Input: part model. Units: mm. Frame: model coordinates. A direction names the side the tool comes from. Coordinates: 2 decimals unless noted, no trailing zeros. Write each loop counter-clockwise with the first axis right and the second up, starting at its lowest first coordinate (ties: lowest second). Pieces come first, ordered by that corner, then holes. Notation, with made-up numbers: (19.25, 36.5) - (57.25, 36.5) arc R24 ccw to (57.25, 53.5) - close; hole circle Ø8 at (55.25, -17). An arc over 180 degrees is marked (long way). One line per question, with ' | ' between items. Start each with the question number.
1) Section query C-C on x = -10. Return loops of the section in (y, z).
2) Section query A-A on x = 0. Return loops of the section in (y, z).
3) Line query: line 1 (X direction, y = -25.95, z = -6.25); line 2 (X direction, y = 10.5, z = 16); line 3 (X direction, y = 39, z = -12.5). Output: solid intervals per line, ascending.
4) Section query B-B on z = 0. Return loops of the section in (x, y), and give its area (3 significant figures).
5) Draft query along X for faces 1 (the flat face through (8.35, 1.67, -7.66)), 2 (the flat face through (-1.4, -25, 11.2)), 3 (the flat face through (0, -28, 0)). Return one class per face: released by +X, released by -X, zero draft, split by the parting line, or undercut.
6) First-contact query: P1, Ø3.5, axis at x = -10, y = 3.5, coming from the +Z side; P2, Ø3, axis at x = 8.5, y = 34, coming from the -Z side; P3, Ø10, axis at y = -17, z = 6, coming from the -X side. Flat tips, straight axial feed; report the tip coordinate or a pass-through.
7) Reachability of faces 4 (the cylindrical face through (0.526, -26.479, 14.169)), 5 (the flat face through (-2.46, -9.28, 13.94)) from +Z, -Z, +X, -X, +Y, -Y: full face, straight path, thin tool, end or side. Return the list, or none.
```python
from build123d import *

# Parameters (mm, degrees)
SKETCH_1_R                  = 20.5
SKETCH_1_R_2                = 17.5
EXTRUDE_1_DEPTH             = 59
CUT_EXTRUDE_1_DEPTH         = 66.738116797
CUT_EXTRUDE_1_DEPTH_BACK    = 66.738116797
EXTRUDE_4_REACH             = 61.536
EXTRUDE_4_DIRECTION_2_REACH = 61.536
EXTRUDE_START               = 28
SKETCH_5_R                  = 20.5
EXTRUDE_5_DEPTH             = 28
CUT_EXTRUDE_6_DEPTH         = 84
SKETCH_15_R                 = 1.75
CUT_EXTRUDE_7_DEPTH         = 83.276971262


with BuildPart() as part:
    # Эскиз1 → Бобышка-Вытянуть1 (new body)
    with BuildSketch(Plane(origin=(0, 0, 0), x_dir=(1, 0, 0), z_dir=(0, 1, 0))):
        with Locations(Location((0, 0, 0), (0, 0, 270))):
            Circle(SKETCH_1_R)
        with Locations(Location((0, 0, 0), (0, 0, 270))):
            Circle(SKETCH_1_R_2, mode=Mode.SUBTRACT)
    extrude(amount=EXTRUDE_1_DEPTH)

    # Эскиз2 → Вырез-Вытянуть1 (cut, two sides: drawn at the far end of the back side and taken through both)
    with BuildSketch(Plane(origin=(0, 0, 0), x_dir=(0, 0, -1), z_dir=(1, 0, 0)).offset(-CUT_EXTRUDE_1_DEPTH_BACK)):
        Polygon((20.5, 59), (-20.5, 59), (-20.5, 11), (20.5, 52), align=None)
    extrude(amount=CUT_EXTRUDE_1_DEPTH + CUT_EXTRUDE_1_DEPTH_BACK, mode=Mode.SUBTRACT)

    # Эскиз3 → Бобышка-Вытянуть4 (add, up to next)
    with BuildSketch(Plane(origin=(0, 0, 0), x_dir=(0, 0, -1), z_dir=(1, 0, 0)), mode=Mode.PRIVATE) as extrude_4_sk1:
        Polygon((-17.5, 1), (17.5, 36), (17.5, 1), (17.5, 0), (-17.5, 0), align=None)
    extrude_4_tool1 = extrude(extrude_4_sk1.sketch, amount=EXTRUDE_4_REACH, mode=Mode.PRIVATE) - part.part
    add(extrude_4_tool1.solids().sort_by_distance((0, 12.009009, -5.518018))[0])

    # Эскиз3 → Бобышка-Вытянуть4 direction 2 (add, up to next)
    with BuildSketch(Plane(origin=(0, 0, 0), x_dir=(0, 0, -1), z_dir=(1, 0, 0)), mode=Mode.PRIVATE) as extrude_4_direction_2_sk1:
        Polygon((-17.5, 1), (17.5, 36), (17.5, 1), (17.5, 0), (-17.5, 0), align=None)
    extrude_4_direction_2_tool1 = extrude(extrude_4_direction_2_sk1.sketch, amount=-EXTRUDE_4_DIRECTION_2_REACH, mode=Mode.PRIVATE) - part.part
    add(extrude_4_direction_2_tool1.solids().sort_by_distance((0, 12.009009, -5.518018))[0])

    # Эскиз5 → Бобышка-Вытянуть5 (add)
    with BuildSketch(Plane.XZ.offset(EXTRUDE_START)):
        with Locations(Location((0, 0, 0), (0, 0, 270))):
            Circle(SKETCH_5_R)
    extrude(amount=-EXTRUDE_5_DEPTH)

    # Эскиз13 → Вырез-Вытянуть6 (cut)
    with BuildSketch(Plane(origin=(0, 59, 0), x_dir=(-1, 0, 0), z_dir=(0, -1, 0))):
        Polygon((7.534421013, 6.25), (9.17986928, 3.4), (12.470765814, 3.4), (14.116214082, 6.25), (12.470765814, 9.1), (9.17986928, 9.1), align=None)
        Polygon((-14.116214082, 6.25), (-12.470765814, 3.4), (-9.17986928, 3.4), (-7.534421013, 6.25), (-9.17986928, 9.1), (-12.470765814, 9.1), align=None)
        Polygon((-3.290896534, -12.5), (-1.645448267, -15.35), (1.645448267, -15.35), (3.290896534, -12.5), (1.645448267, -9.65), (-1.645448267, -9.65), align=None)
    extrude(amount=CUT_EXTRUDE_6_DEPTH, mode=Mode.SUBTRACT)

    # Эскиз15 → Вырез-Вытянуть7 (cut, through all)
    with BuildSketch(Plane(origin=(0, -25, 0), x_dir=(1, 0, 0), z_dir=(0, 1, 0))):
        with Locations(Location((10.825317547, 6.25, 0), (0, 0, 270))):
            Circle(SKETCH_15_R)
        with Locations(Location((-10.825317547, 6.25, 0), (0, 0, 270))):
            Circle(SKETCH_15_R)
        with Locations(Location((0, -12.5, 0), (0, 0, 270))):
            Circle(SKETCH_15_R)
    extrude(amount=-CUT_EXTRUDE_7_DEPTH, mode=Mode.SUBTRACT)


solid = part.part
```
Answer key:
1) outline: (-28, -17.9) - (49.4, -17.9) - (45.86, -14.36) - (32.86, -14.36) - (27.6, -9.1) - (-25, -9.1) - (-25, -7.79) - (-28, -7.79) - close; (-28, -4.71) - (-25, -4.71) - (-25, -3.4) - (21.9, -3.4) - (4.14, 14.36) - (17.14, 14.36) - (13.6, 17.9) - (-28, 17.9) - close
2) outline: (-28, -20.5) - (52, -20.5) - (49, -17.5) - (36, -17.5) - (8.85, 9.65) - (-25, 9.65) - (-25, 10.75) - (-28, 10.75) - close; (-28, 14.25) - (-25, 14.25) - (-25, 15.35) - (3.15, 15.35) - (1, 17.5) - (14, 17.5) - (11, 20.5) - (-28, 20.5) - close
3) line 1: -19.52 to -12.58, -9.08 to 9.08, 12.58 to 19.52 | line 2: -12.82 to -7.09, 7.09 to 12.82 | line 3: -16.25 to -12.25, 12.25 to 16.25
4) outline: (-20.5, -28) - (20.5, -28) - (20.5, 31.5) - (17.5, 31.5) - (17.5, 18.5) - (-17.5, 18.5) - (-17.5, 31.5) - (-20.5, 31.5) - close | area: 1,980 mm²
5) face 1: undercut | face 2: undercut | face 3: zero draft
6) P1: z = 18.77 | P2: z = -19.27 | P3: x = -20.48
7) face 4: +Y, -Y | face 5: +Y
